Can you work these out from the model? Positions are in its coordinate system, mm. Face numbers are marked on the shaded views. A direction names the side the tool comes from. Round coordinates to 2 decimals unless told otherwise and drop trailing zeros. Order: outer loops, then holes, each group sorted by start corner. A loop starts at its lowest first (then second) coordinate and runs counter-clockwise, first axis right, second up. Notation, with made-up numbers: (36.5, -36) - (48.5, -36) arc R19 cw to (48.5, -22) - close; hole circle Ø4 at (25, 44.5). An arc over 180 degrees is marked (long way). Write item = value, one per line.
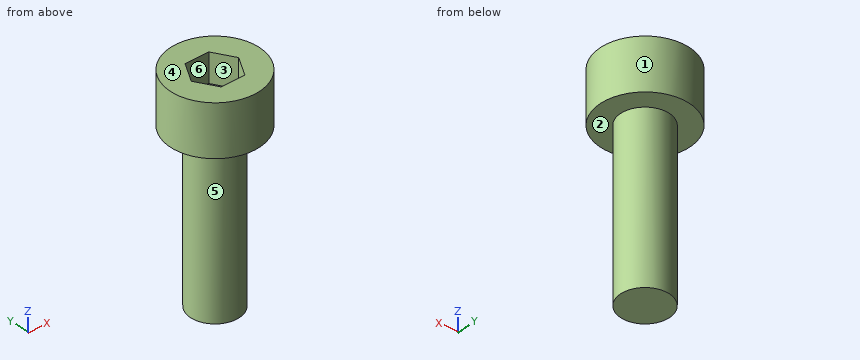
Solid Edge part; units mm, degrees
sketch "Sketch1" plane through (0, 0, 0) normal (0, 0, 1) x (1, 0, 0)
  circle A0 centre (0, 0) radius 2.7
extrude "Protrusion1" add sketch "Sketch1" along normal blind 3.1
sketch "Sketch2" plane through (0, 0, 3.1) normal (0, 0, 1) x (1, 0, 0)
  line L0 (-1.4434, 0) -> (-0.7217, -1.25)
  line L1 (-0.7217, -1.25) -> (0.7217, -1.25)
  line L2 (0.7217, -1.25) -> (1.4434, 0)
  line L3 (1.4434, 0) -> (0.7217, 1.25)
  line L4 (0.7217, 1.25) -> (-0.7217, 1.25)
  line L5 (-0.7217, 1.25) -> (-1.4434, 0)
extrude "ExtrudedCutout_1" cut sketch "Sketch2" against normal blind 1.75
sketch "Sketch3" plane through (0, 0, 0) normal (0, 0, -1) x (1, 0, 0)
  circle A0 centre (0, 0) radius 1.475
extrude "ExtrudedProtrusion_2" add sketch "Sketch3" along normal blind 10
(1) If we section it at B-B (x = 0): Write out the boundary of the cut face in (y, z) (3 decimals).
Computed:
outline = (-2.7, 0) - (-1.475, 0) - (-1.475, -10) - (1.475, -10) - (1.475, 0) - (2.7, 0) - (2.7, 3.1) - (1.25, 3.1) - (1.25, 1.35) - (-1.25, 1.35) - (-1.25, 3.1) - (-2.7, 3.1) - close
(2) If we section it at D-D (y = -1.8): Write out the boundary of the cut face in (x, z), plus the area to 3 significant figures.
Computed:
outline = (-2.01, 0) - (2.01, 0) - (2.01, 3.1) - (-2.01, 3.1) - close
area = 12.5 mm^2
(3) Will these pins go through, and if not, where does the flat tip stop? P1, Ø2, axis at x = 0.5, z = 0.5, coming from the +Y side; P2, Ø2, axis at x = -1.5, z = 1, coming from the -Y side; P3, Ø2, axis at x = 0, y = 0, coming from the +Z side; P4, Ø2, axis at y = -1.5, z = -7, coming from the -X side.
Computed:
P1 = 2.7
P2 = -2.65
P3 = 1.35
P4 = -1.39
(4) If we section it at C-C (z = 0.5): Write out the boundary of the cut face in (x, y).
Computed:
outline = circle Ø5.4 at (0, 0)
(5) If we section it at A-A (z = 2.25): Write out the boundary of the cut face in (x, y), plus the area to 3 significant figures.
Computed:
outline = circle Ø5.4 at (0, 0); hole (-1.44, 0) - (-0.72, -1.25) - (0.72, -1.25) - (1.44, 0) - (0.72, 1.25) - (-0.72, 1.25) - close
area = 17.5 mm^2
(6) If I drill on line 1 (Z direction, x = -0.75, y = -1.95); line 2 (Z direction, x = -0.35, y = 1.05); line 3 (Y direction, x = -0.75, z = -4), over which ranges is the centre line in solid material (lowest first)? Write a range as from..to.
Computed:
line_1 = 0..3.1
line_2 = -10..1.35
line_3 = -1.27..1.27
(7) Thinking about a two-plate mould opening in Y: for the marked faces 1, 2 and 3, which applies, +Y half, -Y half, draft (parallel to the pull), parting line (faces both ways), or undercut?
Computed:
face_1 = parting line
face_2 = draft
face_3 = undercut
(8) On a 3-axis mill with a long thin cutter (end or side, diameter ignored), from which of +Z, -Z, +X, -X, +Y, -Y can I reach the whole of each face in a straight line? I mean the marked faces 4, 5 and 6. Say none if no direction works.
Computed:
face_4 = +Z, +X, -X, +Y, -Y
face_5 = -Z
face_6 = +Z
